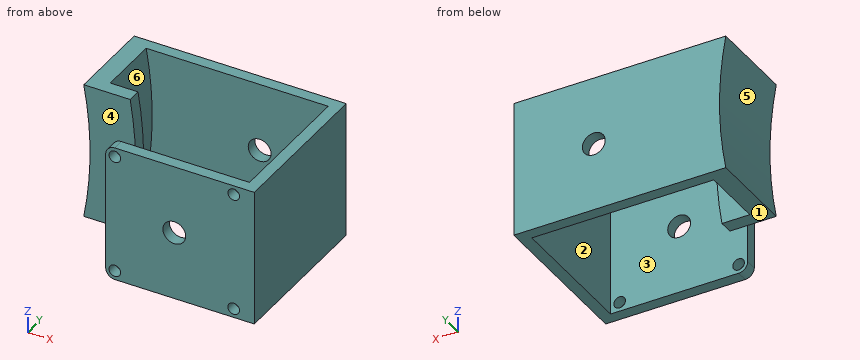
from build123d import *

# Parameters (mm, degrees)
SKETCH1_R           = 2.55
BOSS_EXTRUDE1_DEPTH = 5
SKETCH2_R           = 5
CUT_EXTRUDE1_DEPTH  = 10
SKETCH3_W           = 5
SKETCH3_H           = 60
BOSS_EXTRUDE2_DEPTH = 70
SKETCH4_W           = 80
SKETCH4_H           = 60
BOSS_EXTRUDE4_DEPTH = 5
SKETCH5_R           = 5
CUT_EXTRUDE3_DEPTH  = 5
BOSS_EXTRUDE6_DEPTH = 6
BOSS_EXTRUDE7_START = -32.4
BOSS_EXTRUDE7_DEPTH = 32.4


# Read off the part's stored shape, not the designer's step: Boss-Extrude7
with BuildPart() as part:
    # Sketch1 → Boss-Extrude1 (new body)
    with BuildSketch(Plane(origin=(0, 0, 0), x_dir=(1, 0, 0), z_dir=(0, 1, 0))):
        with BuildLine():
            Line((-26, -30), (30, -30))
            Line((30, -30), (30, 30))
            Line((30, 30), (-26, 30))
            ThreePointArc((-26, 30), (-28.828427125, 28.828427125), (-30, 26))
            Line((-30, 26), (-30, -26))
            ThreePointArc((-30, -26), (-28.828427125, -28.828427125), (-26, -30))
        make_face()
        with Locations(Location((26, 26, 0), (0, 0, 270))):
            Circle(SKETCH1_R, mode=Mode.SUBTRACT)
        with Locations(Location((-26, 26, 0), (0, 0, 270))):
            Circle(SKETCH1_R, mode=Mode.SUBTRACT)
        with Locations(Location((-26, -26, 0), (0, 0, 270))):
            Circle(SKETCH1_R, mode=Mode.SUBTRACT)
        with Locations(Location((26, -26, 0), (0, 0, 270))):
            Circle(SKETCH1_R, mode=Mode.SUBTRACT)
    extrude(amount=BOSS_EXTRUDE1_DEPTH)

    # Sketch2 → Cut-Extrude1 (cut)
    with BuildSketch(Plane(origin=(0, 5, 0), x_dir=(1, 0, 0), z_dir=(0, 1, 0))):
        with Locations(Location((0, 0, 0), (0, 0, 270))):
            Circle(SKETCH2_R)
    extrude(amount=-CUT_EXTRUDE1_DEPTH, mode=Mode.SUBTRACT)

    # Sketch3 → Boss-Extrude2 (add)
    with BuildSketch(Plane.XZ):
        with Locations((32.5, 0)):
            Rectangle(SKETCH3_W, SKETCH3_H)
    extrude(amount=-BOSS_EXTRUDE2_DEPTH)

    # Sketch4 → Boss-Extrude4 (add)
    with BuildSketch(Plane(origin=(0, 70, 0), x_dir=(1, 0, 0), z_dir=(0, 1, 0))):
        with Locations((-10, 0)):
            Rectangle(SKETCH4_W, SKETCH4_H)
    extrude(amount=-BOSS_EXTRUDE4_DEPTH)

    # Sketch5 → Cut-Extrude3 (cut)
    with BuildSketch(Plane(origin=(0, 70, 0), x_dir=(1, 0, 0), z_dir=(0, 1, 0))):
        with Locations(Location((0, 0, 0), (0, 0, 270))):
            Circle(SKETCH5_R)
    extrude(amount=-CUT_EXTRUDE3_DEPTH, mode=Mode.SUBTRACT)



with BuildPart() as body_2:
    # Sketch10 → Boss-Extrude6 (new body)
    with BuildSketch(Plane(origin=(0, 31.6, 0), x_dir=(1, 0, 0), z_dir=(0, 1, 0))):
        with BuildLine():
            Line((-37.448637365, -30), (-57.750192604, -30))
            ThreePointArc((-57.750192604, -30), (-55, 0), (-57.750192604, 30))
            Line((-57.750192604, 30), (-37.448637365, 30))
            ThreePointArc((-37.448637365, 30), (-35, 0), (-37.448637365, -30))
        make_face()
    extrude(amount=BOSS_EXTRUDE6_DEPTH)


with BuildPart() as part_1:
    add(part.part)

    add(body_2.part)  # Boss-Extrude7 merges body 2
    # Boss-Extrude7 outline → Boss-Extrude7 (add)
    with BuildSketch(Plane(origin=(0, 70, 0), x_dir=(1, 0, 0), z_dir=(0, 1, 0)).offset(BOSS_EXTRUDE7_START)):
        with BuildLine():
            ThreePointArc((-57.750192604, 30), (-55, 0), (-57.750192604, -30))
            Line((-57.750192604, -30), (-49.621010685, -30))
            ThreePointArc((-49.621010685, -30), (-47, 0), (-49.621010685, 30))
            Line((-49.621010685, 30), (-57.750192604, 30))
        make_face()
    extrude(amount=BOSS_EXTRUDE7_DEPTH)


solid = part_1.part
Model file for the job. Use its own axes, mm. Face numbers are marked on the shaded views. A direction names the side the tool comes from. Give positions to 0.01 mm unless a question says otherwise; leave off trailing zeros. Loops run counter-clockwise (first coordinate to the right, second up) from the corner with the lowest first, then second, coordinate; pieces in that order, holes last. Notation, with made-up numbers: (71.5, 40.25) - (114.5, 40.25) arc R19 ccw to (114.5, 60.25) - close; hole circle Ø8 at (44.5, -33). An arc over 180 degrees is marked (long way). Use one line per item in the form item = value.
(1) Cut at B-B (x = -38.5). Give the cut face in (y, z).
Determined:
outline = (31.6, -30) - (37.6, -30) - (37.6, 30) - (31.6, 30) - close; (65, -30) - (70, -30) - (70, 30) - (65, 30) - close
(2) Drop flat-ended pins along their axis: P1, Ø1, axis at x = -24, z = 23.5, coming from the -Y side; P2, Ø10, axis at y = 41.5, z = 2.5, coming from the -X side; P3, Ø5.5, axis at y = 3, z = 0.5, coming from the -X side; P4, Ø11.5, axis at x = -51.5, z = 2.5, coming from the -Y side. Give the stop position or say it passes through.
Determined:
P1 = 0
P2 = -55.17
P3 = -30
P4 = 31.6
(3) Drill centre lines: L1, parallel to X at y = 3.65, z = 26; L2, parallel to Y at x = -6, z = -14; L3, parallel to X at y = 67.15, z = 0. Where is each one in solid material? Low to high.
Determined:
L1 = -30 to -28.55, -23.45 to 23.45, 28.55 to 35
L2 = 0 to 5, 65 to 70
L3 = -55 to -5, 5 to 35
(4) Cut at C-C (y = 50.5). Give the cut face in (x, z), then the cut area to 3 significant figures.
Determined:
outline = (-57.75, -30) - (-49.62, -30) arc R173 ccw to (-49.62, 30) - (-57.75, 30) arc R165 cw to start; (30, -30) - (35, -30) - (35, 30) - (30, 30) - close
area = 783 mm^2
(5) Cut at D-D (z = 15). Give the cut face in (x, y).
Determined:
outline = (-55.68, 31.6) - (-35.61, 31.6) - (-35.61, 37.6) - (-47.65, 37.6) - (-47.65, 65) - (30, 65) - (30, 5) - (-30, 5) - (-30, 0) - (35, 0) - (35, 70) - (-55.68, 70) - close
(6) Cut at A-A (x = 26). Give the cut face in (y, z).
Determined:
outline = (0, -30) - (5, -30) - (5, -28.55) - (0, -28.55) - close; (0, -23.45) - (5, -23.45) - (5, 23.45) - (0, 23.45) - close; (0, 28.55) - (5, 28.55) - (5, 30) - (0, 30) - close; (65, -30) - (70, -30) - (70, 30) - (65, 30) - close
(7) 3-axis set-ups, long thin cutter, end or side, ignore diameter. For the marked faces 1, 2 and 3: which of +Z, -Z, +X, -X, +Y, -Y reach the whole face in a straight line?
Determined:
face_1 = -Z, +X, -X, +Y, -Y
face_2 = +Z, -Z
face_3 = +Z, -Z, -X
(8) Pull direction Y, two halves, no side cores. Call the marked faces 4, 5 and 6: pulls with the +Y half, pulls with the -Y half, needs draft (parallel to the pull), parting line crosses it, or undercut.
Determined:
face_4 = pulls with the -Y half
face_5 = needs draft
face_6 = undercut
